Check sheet for the modelled part. Datum: model origin and axes. Units: mm. A direction names the side the tool comes from. Coordinates: 2 decimals unless noted, no trailing zeros. Order: outer loops, then holes, each group sorted by start corner. A loop starts at its lowest first (then second) coordinate and runs counter-clockwise, first axis right, second up.
1. Cross-section at A-A (x = 0). Enter the section's corners in (y, z), then the cut area to 4 significant figures.
2. Set-up check for faces 1 (the flat face through (-7, -6, 6)), 2 (the cylindrical face through (-0.51, -4.62, -11.46)): record each of +Z, -Z, +X, -X, +Y, -Y from which the full face is reachable in a straight line by a thin tool's end or side.
3. Thickness scan on line 1 (Y direction, x = 0, z = -10.5); line 2 (Z direction, x = 0, y = -3.95); line 3 (X direction, y = -3.85, z = 0). Record the ranges inside material, lowest first.
4. Cross-section at B-B (z = -11.5). Enter the section's corners in (x, y), then the cut area to 3 significant figures.
5. Cross-section at D-D (y = -0.5). Enter the section's corners in (x, z).
6. Gauge pin test, flat ends, axial feed: pin 1 Ø1.5 at (x, y) = (-1.5, -2) entering from -Z; pin 2 Ø2 at (x, y) = (5.5, -4) entering from +Z; pin 3 Ø3 at (x, y) = (8, -4.5) entering from +Z. Record the tip position at first contact, or that the pin passes through.
7. Cross-section at C-C (y = -3). Enter the section's corners in (x, z).
8. Draft check along Z on faces 3 (the cylindrical face through (-1.84, -2.71, 8.3)), 4 (the flat face through (6.2, 0, 6.2)), 5 (the cylindrical face through (6.691, -3.042, -12.864)). Enter one of: released by +Z, released by -Z, zero draft, split by the parting line, or undercut.
Autodesk Inventor part; units mm, degrees
ref_plane "YZ Plane" through (0, 0, 0) normal (1, 0, 0) x (0, 1, 0)
ref_plane "XZ Plane" through (0, 0, 0) normal (0, 1, 0) x (-1, 0, 0)
ref_plane "XY Plane" through (0, 0, 0) normal (0, 0, 1) x (1, 0, 0)
sketch "Sketch1" plane through (0, 0, 0) normal (0, 0, 1) x (1, 0, 0)
  line L0 (8.5, 0) -> (14.5, 0)
  line L1 (14.5, 0) -> (14.5, 2.5)
  line L2 (14.5, 2.5) -> (8.5, 2.5)
  line L3 (8.5, 2.5) -> (8.5, 0)
  line L4 (8.5, 0) -> (14.5, 0)
  line L5 (14.5, 0) -> (14.5, -6)
  line L6 (14.5, -6) -> (8.5, -6)
  line L7 (8.5, -6) -> (8.5, 0)
  line L8 (0, -7.7) -> (0, 4.2)
  point P0 (0, 0)
  point P1 (14.5, 0)
  dimension "d0" = 2.5
  dimension "d1" = 8.5
  dimension "d2" = 6
  dimension "d3" = 6
  dimension "d4" = 6
revolve "Revolution1" add sketch "Sketch1" angle 360 about axis through (0, -10, 0) along (0, 1, 0) contours L0 L5 L6 L7
sketch "Sketch2" plane through (0, 0, 0) normal (0, 0, 1) x (1, 0, 0)
  line L0 (0, 0) -> (0, -6) construction
  line L1 (8.5, -6) -> (-8.5, -6)
  line L2 (8.5, 0) -> (-8.5, 0)
  point P0 (0, -3)
hole "Hole1" at (0, -3, 0) direction (0, 0, -1) diameter 3.4 end through all
chamfer "Chamfer1" distance 0.5 angle 45 1 edges at (-8.5, -6, 0)
properties part number "spring safety"
Data:
1. outline: (-6, -14.5) - (-4.7, -14.5) - (-4.7, -8.5) - (-5.5, -8.5) - (-6, -9) - close; (-6, 9) - (-5.5, 8.5) - (0, 8.5) - (0, 14.5) - (-6, 14.5) - close; (-1.3, -14.5) - (0, -14.5) - (0, -8.5) - (-1.3, -8.5) - close
1. area: 51.35 mm2
2. face 1: +Z, -Z, +X, -X, -Y
2. face 2: -Z
3. line 1: y = -6 to -4.7, -1.3 to 0
3. line 2: z = 8.5 to 14.5
3. line 3: x = -14.5 to -8.5, 8.5 to 14.5
4. outline: (-8.83, -6) - (8.83, -6) - (8.83, 0) - (-8.83, 0) - close; hole circle Ø3.4 at (0, -3)
4. area: 96.9 mm2
5. outline: circle Ø29 at (0, 0); hole circle Ø17 at (0, 0)
6. pin 1: stops at z = -14.47
6. pin 2: stops at z = 13.78
6. pin 3: stops at z = 12.96
7. outline: (-1.7, -14.4) - (-1.7, -8.33) arc R8.5 cw (long way) to (1.7, -8.33) - (1.7, -14.4) arc R14.5 ccw (long way) to start
8. face 3: undercut
8. face 4: zero draft
8. face 5: split by the parting line
